Geometry: final body of the model. Coordinates: model frame, mm. A direction names the side the tool comes from. Round coordinates to 2 decimals unless told otherwise and drop trailing zeros. Order: outer loops, then holes, each group sorted by start corner. A loop starts at its lowest first (then second) coordinate and runs counter-clockwise, first axis right, second up. Notation, with made-up numbers: M 16,73.5 L 31,73.5 A18 ccw 31,92.5 Z; hole C 38.5,36 d5. An arc over 180 degrees is marked long. Put each result on its own line as item: value. Start each with the question number.
1) Material intervals for probe 1 along Y at (x, z) = (68, 1.35); probe 2 along Y at (x, z) = (239.5, 2.4); probe 3 along X at (y, z) = (6.25, 2), sorted ascending. Write a range as [from, to].
2) First-contact query: P1, Ø1.9, axis at x = 0, y = 5.9, coming from the +Z side. Flat tip, straight axial feed; report the tip coordinate or a pass-through.
3) Section A-A, the plane z = 0.65. Count the separate pieces of the cut face and the enclosed holes in it, then the cut area to 3 significant figures.
4) Section B-B, the plane x = 133.5. Return loops of the section in (y, z).
5) Access query for faces 1 (the flat face through (133, 5.9, 2)), 2 (the flat face through (0, 8.95, 2)), 3 (the flat face through (136, 0, 2)). Directions: +Z, -Z, +X, -X, +Y, -Y. A direction counts if a zero-diameter tool reaches every point of the face in a straight line with its end or side. Return the directions, or none.
Autodesk Inventor part; units mm, degrees
ref_plane "YZ Plane" through (0, 0, 0) normal (1, 0, 0) x (0, 1, 0)
ref_plane "XZ Plane" through (0, 0, 0) normal (0, 1, 0) x (-1, 0, 0)
ref_plane "XY Plane" through (0, 0, 0) normal (0, 0, 1) x (1, 0, 0)
sketch "Sketch1" plane through (0, 0, 0) normal (0, 0, 1) x (1, 0, 0)
  circle A0 centre (0, 0) radius 1.05
  circle A1 centre (0, 5.9) radius 1.05
  line L0 (-3, 8.95) -> (3, 8.95)
  line L1 (3, 8.95) -> (3, -3.05)
  line L2 (3, -3.05) -> (-3, -3.05)
  line L3 (-3, -3.05) -> (-3, 8.95)
  line L4 (3, 5.9) -> (263, 5.9)
  line L5 (263, 5.9) -> (263, 0)
  line L6 (263, 0) -> (3, 0)
  line L7 (3, 0) -> (3, 5.9)
  point P0 (3, 0)
  dimension "d0" = 2.1
  dimension "d1" = 2.1
  dimension "d2" = 5.9
  dimension "d3" = 3
  dimension "d4" = 3
  dimension "d5" = 12
  dimension "d6" = 3.05
  dimension "d7" = 260
extrude "Extrusion1" add sketch "Sketch1" along normal blind 4
sketch "Sketch2" plane through (0, 0, 4) normal (0, 0, 1) x (1, 0, 0)
  circle A0 centre (8, 2.95) radius 1
  line L0 (-3, 8.95) -> (-3, -3.05)
  line L1 (3, 5.9) -> (3, 8.95)
  point P0 (0, 0)
  point P1 (-3, 2.95)
  dimension "d10" = 2
  dimension "d11" = 5
extrude "Extrusion2" cut sketch "Sketch2" against normal blind 10
pattern_linear "Rectangular Pattern1" count 26 spacing 10 along (1, 0, 0) of "Extrusion2"
chamfer "Chamfer1" distance 3 angle 45 2 edges at (3, 5.9, 2) (3, 0, 2)
properties part number "Test_feather"
Result sheet:
1. probe 1: y = [0, 1.95], [3.95, 5.9]
1. probe 2: y = [0, 5.9]
1. probe 3: x = [-3, -0.99], [0.99, 5.65]
2. P1: passes through
3. separate pieces: 1
3. enclosed holes: 28
3. area: 1,530 mm2
4. outline: M 0,0 L 5.9,0 L 5.9,4 L 0,4 Z
5. face 1: +Z, -Z, +X, +Y
5. face 2: +Z, -Z, +X, -X, +Y
5. face 3: +Z, -Z, +X, -Y
